Autodesk Inventor part; units mm, degrees
ref_plane "YZ Plane" through (0, 0, 0) normal (1, 0, 0) x (0, 1, 0)
ref_plane "XZ Plane" through (0, 0, 0) normal (0, 1, 0) x (-1, 0, 0)
ref_plane "XY Plane" through (0, 0, 0) normal (0, 0, 1) x (1, 0, 0)
sketch "Sketch1" plane through (0, 0, 0) normal (0, 0, 1) x (1, 0, 0)
  line L0 (-11.214, 10.6272) -> (138.786, 10.6272)
  line L1 (138.786, 10.6272) -> (138.786, -139.3728)
  line L2 (138.786, -139.3728) -> (-11.214, -139.3728)
  line L3 (-11.214, -139.3728) -> (-11.214, 10.6272)
  point P0 (0, 0)
  dimension "d0" = 150
  dimension "d1" = 150
ref_plane "Work Plane2" through (-11.214, 10.6272, -6.35) normal (0, 0, -1) x (1, 0, 0)
ref_plane "Work Plane1" through (-11.214, 10.6272, 0) normal (0, 0, -1) x (1, 0, 0)
sketch "Sketch2" plane through (-11.214, 10.6272, -6.35) normal (0, 0, -1) x (1, 0, 0)
  line L0 (143.6624, 6.35) -> (6.3624, 6.35)
  line L1 (6.3624, 6.35) -> (6.3624, 143.65)
  line L2 (6.3624, 143.65) -> (143.6624, 143.65)
  line L3 (143.6624, 143.65) -> (143.6624, 6.35)
  line L4 (150, 0) -> (0, 0) construction
  line L5 (0, 0) -> (0, 150) construction
  point P0 (11.214, 10.6272)
  dimension "d3" = 137.3
  dimension "d4" = 137.3
  dimension "d6" = 6.35
  dimension "d7" = 143.6624
loft "Loft1" add profiles "Sketch1", "Sketch2"
sketch "Sketch3" plane through (-11.214, 10.6272, 0) normal (0, 0, 1) x (1, 0, 0)
  line L0 (0, 0) -> (6.3624, -6.35)
  line L1 (150, 0) -> (150, -150)
  line L2 (0, 0) -> (150, -150) construction
  line L3 (0, -150) -> (6.3624, -143.65)
  line L4 (0, -150) -> (150, 0) construction
  circle A0 centre (75, -75) radius 6.35
  point P0 (11.214, -10.6272)
  dimension "d12" = 12.7
extrude "Extrusion1" cut sketch "Sketch3" against normal blind 25.4
properties part number "insulationlid"
For this review, take the finished solid that the model builds, in its own axes (mm). Round coordinates to 2 decimals unless told otherwise and drop trailing zeros. Use a Markdown table: item, result. Add a question column.
Item 1: Insertion check: pin 1 (1.5 mm diameter, centred on x = 82.5, z = -2.5, fed in from +Y); pin 2 (1 mm diameter, centred on y = -105, z = -2, fed in from +X). Each pin has a flat end and moves straight along its axis. Give the tip position at first contact, or say it passes through.
Item 2: To check wall thickness, follow line 1 along Y through (x, z) = (67, -1.75); line 2 along X through (y, z) = (-71, -2.5); line 3 along X through (y, z) = (-47, -5). State the ranges of each line that lie inside material, in increasing order.
Item 3: Mouldability with a two-part tool opening along X and no side actions: class faces 1 (the cylindrical face through (66.716, -70.006, -3.131)), 2 (the flat face through (47, -46, 0)) as released by +X, released by -X, zero draft, split by the parting line, or undercut.
Geometry results:
| question | item | result |
|---|---|---|
| 1 | pin 1 | stops at y = 8.88 |
| 1 | pin 2 | stops at x = 137.29 |
| 2 | line 1 | y = -137.62 to -69.85, -58.9 to 8.88 |
| 2 | line 2 | x = -8.71 to 136.29 |
| 2 | line 3 | x = -6.2 to 133.8 |
| 3 | face 1 | undercut |
| 3 | face 2 | zero draft |
